Geometry: final body of the model. Coordinates: model frame, mm. A direction names the side the tool comes from. Give positions to 0.01 mm unless a question says otherwise; leave off trailing zeros. Order: outer loops, then holes, each group sorted by start corner. A loop starts at its lowest first (then second) coordinate and runs counter-clockwise, first axis right, second up. Notation, with made-up numbers: (19.5, 39) - (69.5, 39) arc R18 ccw to (69.5, 67) - close; hole circle Ø1 at (31.5, -9.75). An arc over 180 degrees is marked (long way). Put each result on its own line as item: value. Start each with the question number.
1. Section B-B on y = 11.75. Return the cut outline in (x, z), plus the area to 3 significant figures.
2. First-contact query: P1, Ø4, axis at x = -13, y = 8.5, coming from the -Z side; P2, Ø3.5, axis at x = -12, y = 10.25, coming from the -Z side; P3, Ø2.5, axis at x = -16.5, y = 10.25, coming from the +Z side; P4, Ø3, axis at x = -1, z = -7, coming from the +Y side. Flat tips, straight axial feed; report the tip coordinate or a pass-through.
3. Ray query, line 1 along X through (y, z) = (-0.3, -8.5); line 2 along Y through (x, z) = (-7.5, -1.1); line 3 along Y through (x, z) = (-12, -1.1). Return the intervals inside material, ascending. Write a range as from..to.
4. Section C-C on x = 3. Return the cut outline in (y, z).
5. Section D-D on z = -5.5. Return the cut outline in (x, y).
6. Mould query, pull axis Y, two halves, no side actions, for faces 3 (the cylindrical face through (-7.039, 9.364, -1.246)), 4 (the flat face through (0, 0, -8)), 5 (the cylindrical face through (5.699, -0.254, -13.215)). Classes: pulls with the +Y half, pulls with the -Y half, needs draft (parallel to the pull), parting line crosses it, or undercut.
7. Section A-A on x = -16.5. Return the cut outline in (y, z), plus the area to 3 significant figures.
8. Set-up query: faces 1 (the flat face through (-7, 8, -1.5)), 2 (the cylindrical face through (-1.99, -0.25, -9.61)). Return all of +Z, -Z, +X, -X, +Y, -Y with unobstructed straight access to the full face (end or side cutting, diameter ignored); none if empty.
from build123d import *

# Parameters (mm, degrees)
SKETCH1_W              = 12
SKETCH1_H              = 27
BASE_FLANGE1_DEPTH     = 0.5
SKETCHED_START         = -6
SKETCHED_BEND1_DEPTH   = 12
SKETCHED_BEND1_2_DEPTH = 12
TAB1_START             = -0.5
TAB1_OUTLINE_W         = 14
TAB1_OUTLINE_H         = 13.751106428
TAB1_DEPTH             = 0.5
SKETCH8_R              = 1
SKETCH8_R_2            = 2
CUT_EXTRUDE1_DEPTH     = 10
SKETCH9_R              = 1.5
CUT_EXTRUDE2_DEPTH     = 10
FILLET1_R              = 1


# Read off the part's stored shape, not the designer's step: Sketched Bend1, Tab1
# Sheet-metal steps are written as plain solids
with BuildPart() as part:
    # Sketch1 → Base-Flange1 (new body)
    with BuildSketch(Plane(origin=(0, 0, 0), x_dir=(1, 0, 0), z_dir=(0, 1, 0))):
        Rectangle(SKETCH1_W, SKETCH1_H)
    extrude(amount=-BASE_FLANGE1_DEPTH)

    # Sketched Bend1 outline → Sketched Bend1 (cut)
    with BuildSketch(Plane.YZ.offset(SKETCHED_START)):
        with BuildLine():
            ThreePointArc((-0.5, -3), (-0.370828693, -2.292893219), (0, -1.677124345))
            Line((0, -1.677124345), (0, 13.5))
            Line((0, 13.5), (-0.5, 13.5))
            Line((-0.5, 13.5), (-0.5, -3))
        make_face()
    extrude(amount=SKETCHED_BEND1_DEPTH, mode=Mode.SUBTRACT)

    # Sketched Bend1 2 outline → Sketched Bend1 2 (add)
    with BuildSketch(Plane.YZ.offset(SKETCHED_START)):
        with BuildLine():
            ThreePointArc((0, -3), (0.439339828, -1.939339828), (1.5, -1.5))
            Line((1.5, -1.5), (15.251106428, -1.5))
            Line((15.251106428, -1.5), (15.251106428, -1))
            Line((15.251106428, -1), (1.5, -1))
            ThreePointArc((1.5, -1), (0.677124344, -1.177124345), (0, -1.677124345))
            Line((0, -1.677124345), (0, -3))
        make_face()
    extrude(amount=SKETCHED_BEND1_2_DEPTH)

    # Tab1 outline → Tab1 (add)
    with BuildSketch(Plane(origin=(0, 0, -1.5), x_dir=(-1, 0, 0), z_dir=(0, 0, -1)).offset(TAB1_START)):
        with Locations((13, 8.375553214)):
            Rectangle(TAB1_OUTLINE_W, TAB1_OUTLINE_H)
    extrude(amount=TAB1_DEPTH)

    # Sketch8 → Cut-Extrude1 (cut)
    with BuildSketch(Plane.XY.offset(-1)):
        with Locations((-16.5, 10.251106428)):
            Circle(SKETCH8_R)
        with Locations((-7.5, 10.251106428)):
            Circle(SKETCH8_R)
        with Locations((-12, 10.251106428)):
            Circle(SKETCH8_R_2)
    extrude(amount=-CUT_EXTRUDE1_DEPTH, mode=Mode.SUBTRACT)

    # Sketch9 → Cut-Extrude2 (cut)
    with BuildSketch(Plane(origin=(0, 0, 0), x_dir=(1, 0, 0), z_dir=(0, 1, 0))):
        with Locations(Location((-3, 8.5, 0), (0, 0, 270))):
            Circle(SKETCH9_R)
        with Locations(Location((3, 8.5, 0), (0, 0, 270))):
            Circle(SKETCH9_R)
    extrude(amount=-CUT_EXTRUDE2_DEPTH, mode=Mode.SUBTRACT)

    # Fillet1
    fillet1_edges = [part.edges().sort_by_distance(p)[0] for p in [
        (-6, -0.25, -13.5),
        (6, -0.25, -13.5),
        (-20, 15.251106428, -1.25),
        (-20, 1.5, -1.25),
        (6, 15.251106428, -1.25),
    ]]
    fillet(fillet1_edges, radius=FILLET1_R)


solid = part.part
Resolved:
1. outline: (-20, -1.5) - (-13.32, -1.5) - (-13.32, -1) - (-20, -1) - close; (-10.68, -1.5) - (6, -1.5) - (6, -1) - (-10.68, -1) - close
1. area: 11.7 mm^2
2. P1: z = -1.5
2. P2: through
2. P3: z = -1
2. P4: y = 0
3. line 1: -6..-4.5, -1.5..1.5, 4.5..6
3. line 2: 1.5..9.25, 11.25..15.25
3. line 3: 1.5..8.25, 12.25..15.25
4. outline: (-0.5, -13.5) - (0, -13.5) - (0, -10) - (-0.5, -10) - close; (-0.5, -7) - (0, -7) - (0, -3) arc R1.5 cw to (1.5, -1.5) - (15.25, -1.5) - (15.25, -1) - (1.5, -1) arc R2 ccw to (-0.5, -3) - close
5. outline: (-6, -0.5) - (6, -0.5) - (6, 0) - (-6, 0) - close
6. face 3: undercut
6. face 4: pulls with the +Y half
6. face 5: needs draft
7. outline: (1.5, -1.5) - (9.25, -1.5) - (9.25, -1) - (1.5, -1) - close; (11.25, -1.5) - (15.25, -1.5) - (15.25, -1) - (11.25, -1) - close
7. area: 5.88 mm^2
8. face 1: -Z, +X, -X, +Y
8. face 2: +Y, -Y
